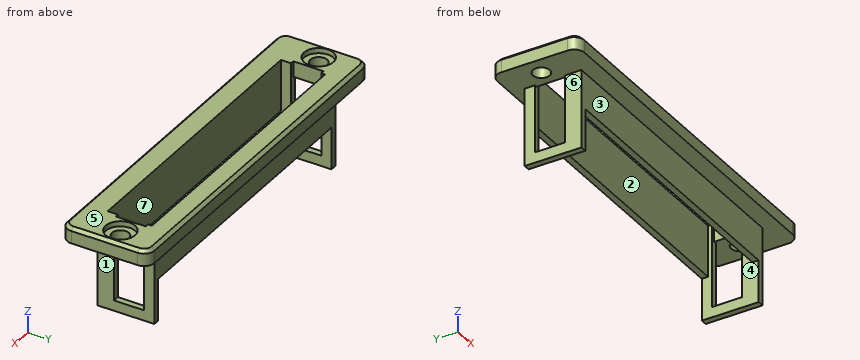
```python
from build123d import *

# Parameters (mm, degrees)
FLANGE_DEPTH             = 3
FRONT_BEVEL_SIZE         = 0.6
OPENING_HOLES_DEPTH      = 36.974236962
OPENING_HOLES_DEPTH_BACK = 36.974236962
SK_OPENING_R             = 1.625
SK_COUNTERBORE_R         = 2.825
COUNTERBORE_DEPTH        = 1
SK_LONG_WALLS_W          = 56.72
SK_LONG_WALLS_H          = 1.2
LONG_WALLS_DEPTH         = 6.9
SK_LEGS_W                = 1.2
SK_LEGS_H                = 1.95
SK_LEGS_H_2              = 3.15
LEGS_DEPTH               = 13
SK_LEG_TIES_W            = 1.2
SK_LEG_TIES_H            = 10.9
LEG_TIES_DEPTH           = 2


with BuildPart() as part:
    # SK Flange → Flange (new body)
    with BuildSketch(Plane.XY):
        with BuildLine():
            Line((-32.635, -9.25), (32.635, -9.25))
            ThreePointArc((32.635, -9.25), (34.049213562, -8.664213562), (34.635, -7.25))
            Line((34.635, -7.25), (34.635, 5.5))
            ThreePointArc((34.635, 5.5), (34.049213562, 6.914213562), (32.635, 7.5))
            Line((32.635, 7.5), (-32.635, 7.5))
            ThreePointArc((-32.635, 7.5), (-34.049213562, 6.914213562), (-34.635, 5.5))
            Line((-34.635, 5.5), (-34.635, -7.25))
            ThreePointArc((-34.635, -7.25), (-34.049213562, -8.664213562), (-32.635, -9.25))
        make_face()
    extrude(amount=FLANGE_DEPTH)

    # Front bevel
    front_bevel_edges = [part.edges().sort_by_distance(p)[0] for p in [
        (34.049213562, -8.664213562, 3),
        (34.635, -0.875, 3),
        (34.049213562, 6.914213562, 3),
        (0, 7.5, 3),
        (-34.049213562, 6.914213562, 3),
        (-34.635, -0.875, 3),
        (-34.049213562, -8.664213562, 3),
        (0, -9.25, 3),
    ]]
    chamfer(front_bevel_edges, length=FRONT_BEVEL_SIZE)

    # SK Opening → Opening + holes (cut, two sides: drawn at the far end of the back side and taken through both)
    with BuildSketch(Plane.XY.offset(-OPENING_HOLES_DEPTH_BACK)):
        with Locations((-31.085, 0)):
            Circle(SK_OPENING_R)
        with Locations((31.085, 0)):
            Circle(SK_OPENING_R)
        Polygon((-27.16, -4.85), (27.16, -4.85), (27.16, -2.9), (27.86, -2.9), (27.86, 2.9), (27.16, 2.9), (27.16, 3.65), (-27.16, 3.65), (-27.16, 2.9), (-27.86, 2.9), (-27.86, -2.9), (-27.16, -2.9), align=None)
    extrude(amount=OPENING_HOLES_DEPTH + OPENING_HOLES_DEPTH_BACK, mode=Mode.SUBTRACT)

    # SK Counterbore → Counterbore (cut)
    with BuildSketch(Plane.XY.offset(3)):
        with Locations((-31.085, 0)):
            Circle(SK_COUNTERBORE_R)
        with Locations((31.085, 0)):
            Circle(SK_COUNTERBORE_R)
    extrude(amount=-COUNTERBORE_DEPTH, mode=Mode.SUBTRACT)

    # SK Long walls → Long walls (add)
    with BuildSketch(Plane.XY):
        with Locations((0, 4.25)):
            Rectangle(SK_LONG_WALLS_W, SK_LONG_WALLS_H)
        with Locations((0, -5.45)):
            Rectangle(SK_LONG_WALLS_W, SK_LONG_WALLS_H)
    extrude(amount=-LONG_WALLS_DEPTH)

    # SK Legs → Legs (add)
    with BuildSketch(Plane.XY):
        with Locations((-27.76, 3.875)):
            Rectangle(SK_LEGS_W, SK_LEGS_H)
        with Locations((-27.76, -4.475)):
            Rectangle(SK_LEGS_W, SK_LEGS_H_2)
        with Locations((27.76, 3.875)):
            Rectangle(SK_LEGS_W, SK_LEGS_H)
        with Locations((27.76, -4.475)):
            Rectangle(SK_LEGS_W, SK_LEGS_H_2)
    extrude(amount=-LEGS_DEPTH)

    # SK Leg ties → Leg ties (add)
    with BuildSketch(Plane.XY.offset(-13)):
        with Locations((-27.76, -0.6)):
            Rectangle(SK_LEG_TIES_W, SK_LEG_TIES_H)
        with Locations((27.76, -0.6)):
            Rectangle(SK_LEG_TIES_W, SK_LEG_TIES_H)
    extrude(amount=-LEG_TIES_DEPTH)


solid = part.part
```
Read the model definition and answer for the solid it produces. Units are mm, in the model's axes. Face numbers are marked on the shaded views. A direction names the side the tool comes from. Coordinates: 2 decimals unless noted, no trailing zeros. Write each loop counter-clockwise with the first axis right and the second up, starting at its lowest first coordinate (ties: lowest second). Pieces come first, ordered by that corner, then holes. Notation, with made-up numbers: (-16.5, 10.25) -> (-5.5, 10.25) arc R27 ccw to (-5.5, 44.25) -> close; hole circle Ø8 at (87, 61.5). An arc over 180 degrees is marked (long way). Return JSON: item names as keys, results as strings.
1. A cutting plane is placed at C-C (y = 0). Give the number of separate pieces and of enclosed holes in the cut face, and give its area (3 significant figures).
Found:
{"separate pieces": "6", "enclosed holes": "0", "area": "20.8 mm2"}
2. A cutting plane is placed at B-B (x = 22.5). Determine the outline of the cut face in (y, z).
Found:
{"outline": "(-9.25, 0) -> (-6.05, 0) -> (-6.05, -6.9) -> (-4.85, -6.9) -> (-4.85, 3) -> (-8.65, 3) -> (-9.25, 2.4) -> close; (3.65, -6.9) -> (4.85, -6.9) -> (4.85, 0) -> (7.5, 0) -> (7.5, 2.4) -> (6.9, 3) -> (3.65, 3) -> close"}
3. A cutting plane is placed at D-D (z = -5.75). Determine the outline of the cut face in (x, y), and give its area (3 significant figures).
Found:
{"outline": "(-28.36, -6.05) -> (28.36, -6.05) -> (28.36, -2.9) -> (27.16, -2.9) -> (27.16, -4.85) -> (-27.16, -4.85) -> (-27.16, -2.9) -> (-28.36, -2.9) -> close; (-28.36, 2.9) -> (-27.16, 2.9) -> (-27.16, 3.65) -> (27.16, 3.65) -> (27.16, 2.9) -> (28.36, 2.9) -> (28.36, 4.85) -> (-28.36, 4.85) -> close", "area": "143 mm2"}
4. Find the intervals of material crossed by line 1 along X through (y, z) = (0, 1.5) (3 decimals); line 2 along Y through (x, z) = (-24, -2.5); line 3 along X through (y, z) = (-5.25, -13.75), in increasing order. Write a range as from..to.
Found:
{"line 1": "-34.635..-32.71, -29.46..-27.86, 27.86..29.46, 32.71..34.635", "line 2": "-6.05..-4.85, 3.65..4.85", "line 3": "-28.36..-27.16, 27.16..28.36"}
5. Each of these flat-tipped pins is pushed along its axis until it touches: P1, Ø3.5, axis at y = -1, z = -2, coming from the +X side; P2, Ø5, axis at x = -26, z = -5.5, coming from the +Y side; P3, Ø1, axis at x = -27.5, z = -6.5, coming from the -Y side; P4, Ø4, axis at x = -31.085, y = 0, coming from the -Z side. Where does it stop, or does it pass through?
Found:
{"P1": "through", "P2": "y = 4.85", "P3": "y = -6.05", "P4": "z = 0"}
6. A cutting plane is placed at A-A (z = -9.25). Determine the outline of the cut face in (x, y).
Found:
{"outline": "(-28.36, -6.05) -> (-27.16, -6.05) -> (-27.16, -2.9) -> (-28.36, -2.9) -> close; (-28.36, 2.9) -> (-27.16, 2.9) -> (-27.16, 4.85) -> (-28.36, 4.85) -> close; (27.16, -6.05) -> (28.36, -6.05) -> (28.36, -2.9) -> (27.16, -2.9) -> close; (27.16, 2.9) -> (28.36, 2.9) -> (28.36, 4.85) -> (27.16, 4.85) -> close"}
7. Determine the mould class of the marked faces 1, 2, 3 and 4 for opening direction Y: pulls with the +Y half, pulls with the -Y half, needs draft (parallel to the pull), parting line crosses it, or undercut.
Found:
{"face 1": "needs draft", "face 2": "undercut", "face 3": "pulls with the -Y half", "face 4": "undercut"}
8. A tool of negligible diameter and unlimited length cuts with its end or side. For the marked faces 5, 6 and 7, from which of +Z, -Z, +X, -X, +Y, -Y can it reach the whole face along a straight path? Write none if from no direction.
Found:
{"face 5": "+Z, +X, -X, +Y, -Y", "face 6": "-Z, -X, +Y, -Y", "face 7": "+Z, -Z"}
